Can you work these out from the model? Positions are in its coordinate system, mm. A direction names the side the tool comes from. Round coordinates to 2 decimals unless told otherwise and drop trailing zeros. Write each loop counter-clockwise with the first axis right and the second up, starting at its lowest first coordinate (ties: lowest second). Pieces come first, ordered by that corner, then holes. Notation, with made-up numbers: (43.25, -35.75) - (60.25, -35.75) arc R30 ccw to (60.25, -6.75) - close; hole circle Ø1 at (9, 22). An arc over 180 degrees is marked (long way). One line per item, written item: value. Start each with the question number.
(1) I want a section at C-C on y = 44. List the corners of the cut face in (x, z) for me, plus the area to 3 significant figures.
(2) I'm going to push flat-ended pins straight in: pin 1 Ø2 at (x, z) = (0, 15.5) entering from +Y; pin 2 Ø3 at (y, z) = (23.5, 0) entering from +X; pin 3 Ø2 at (x, y) = (-5, 17) entering from +Z. Where does each tip first touch, or does it pass through?
(3) If I drill on L1, parallel to Z at x = 0, y = 48.75; L2, parallel to Z at x = 1, y = 15.5; L3, parallel to Y at x = 0.5, z = -3, over which ranges is the centre line in solid material (lowest first)? Write a range as from..to.
(4) I want a section at A-A on y = 33. List the corners of the cut face in (x, z) for me, plus the area to 3 significant figures.
(5) I want a section at D-D on x = 0. Give the number of separate pieces and of enclosed holes in the cut face, plus the area to 3 significant figures.
(6) On a 3-axis mill with a long thin cutter (end or side, diameter ignored), from which of +Z, -Z, +X, -X, +Y, -Y can I reach the whole of each face in a straight line? I mean faces 1 (the face through (0, 43, 16)), 2 (the face through (0, 50, 0)), 3 (the face through (0, 33, -17.2)). Say none if no direction works.
(7) Thinking about a two-plate mould opening in Z: for faces 4 (the face through (-6.5, 25, -4)), 5 (the face through (0, 25, -22)), 6 (the face through (0, 7, -16)), which applies, +Z half, -Z half, draft (parallel to the pull), parting line (faces both ways), or undercut?
(8) I want a section at B-B on z = 0. List the corners of the cut face in (x, y) for me (3 decimals), plus the area to 3 significant figures.
Autodesk Inventor part; units mm, degrees
ref_plane "YZ Plane" through (0, 0, 0) normal (1, 0, 0) x (0, 1, 0)
ref_plane "XZ Plane" through (0, 0, 0) normal (0, 1, 0) x (-1, 0, 0)
ref_plane "XY Plane" through (0, 0, 0) normal (0, 0, 1) x (1, 0, 0)
sketch "Эскиз1" plane through (0, 0, 0) normal (0, 1, 0) x (-1, 0, 0)
  line L0 (6.5, 31) -> (-6.5, 31)
  line L1 (-6.5, 31) -> (-6.5, -31)
  line L2 (-6.5, -31) -> (6.5, -31)
  line L3 (6.5, -31) -> (6.5, 31)
  line L4 (-6.5, 31) -> (6.5, -31) construction
  line L5 (0, 31) -> (0, -31) construction
  circle A0 centre (0, 16) radius 2
  line L6 (6.5, 0) -> (-6.5, 0) construction
  circle A1 centre (0, -16) radius 2
  point P0 (0, 0)
  point P1 (0, 0)
  dimension "d0" = 13
  dimension "d1" = 62
  dimension "d2" = 16
  dimension "d3" = 4
extrude "Выдавливание1" add sketch "Эскиз1" along normal blind 32
sketch "Эскиз2" plane through (6.5, 0, 31) normal (1, 0, 0) x (0, 0, -1)
  line L0 (0, 32) -> (62, 32)
  line L1 (62, 0) -> (0, 0)
  line L2 (62, 32) -> (0, 0) construction
  circle A0 centre (31, 16) radius 10.15
  line L3 (20.85, 16) -> (41.15, 16) construction
  circle A1 centre (31, 16) radius 10.125
  line L4 (31, 26.125) -> (31, 5.875)
  line L5 (62, 0) -> (62, 32)
  circle A2 centre (31, 16) radius 5
  line L6 (31, 16) -> (24.504809, 12.25) construction
  line L7 (31, 16) -> (37.495191, 12.25) construction
  circle A3 centre (31, 16) radius 7.5 construction
  circle A4 centre (31, 23.5) radius 1.3
  circle A5 centre (37.495191, 12.25) radius 1.3
  circle A6 centre (24.504809, 12.25) radius 1.3
  line L8 (37.495191, 12.25) -> (36.55555, 10.622495) construction
  circle A7 centre (31, 16) radius 10 construction
  line L9 (37.495191, 12.25) -> (39.660254, 11) construction
  point P0 (31, 0)
  dimension "d60" = 20
  dimension "d9" = 20.3
  dimension "d17" = 10
  dimension "d21" = 20.25
  dimension "d57" = 120
  dimension "d58" = 120
  dimension "d59" = 2.6
  dimension "d61" = 2.5
  dimension "d65" = 15
extrude "Выдавливание3" cut sketch "Эскиз2" against normal through all contours A4 L4 | L4 A4 | A2 L4 | L4 A2 | A5 | A6
sketch "Эскиз2 outline for Выдавливание4" plane through (6.5, 0, 31) normal (1, 0, 0) x (0, 0, -1)
  circle A0 centre (31, 16) radius 10.125
extrude "Выдавливание4" cut sketch "Эскиз2 outline for Выдавливание4" against normal blind 9
sketch "Эскиз3" plane through (0, 32, 0) normal (0, 1, 0) x (1, 0, 0)
  circle A0 centre (0, -16) radius 2
  circle A1 centre (0, 16) radius 2
  point P0 (0, 0)
extrude "Выдавливание5" add sketch "Эскиз3" against normal blind 25
fillet "Сопряжение1" radius 6 2 edges at (6.5, 16, 31) (6.5, 16, -31)
chamfer "Фаска1" distance 1.3 angle 45 3 edges at (-6.5, 12.25, 7.7952) (-6.5, 12.25, -5.1952) (-6.5, 23.5, 1.3)
sketch "Эскиз6" plane through (0, 32, 0) normal (0, 1, 0) x (1, 0, 0)
  arc A0 (6.5, 25) -> (0.5, 31) centre (0.5, 25) ccw
  line L0 (0.5, 31) -> (-6.5, 31)
  line L1 (-6.5, 31) -> (-6.5, -31)
  line L2 (-6.5, -31) -> (0.5, -31)
  arc A1 (0.5, -31) -> (6.5, -25) centre (0.5, -25) ccw
  line L3 (6.5, -25) -> (6.5, 25)
  point P0 (0, 0)
extrude "Выдавливание6" add sketch "Эскиз6" along normal blind 18
sketch "Эскиз7" plane through (0, 50, 0) normal (0, 1, 0) x (1, 0, 0)
  circle A0 centre (0, -16) radius 2
  circle A1 centre (0, 16) radius 2
  point P0 (0, 0)
extrude "Выдавливание7" cut sketch "Эскиз7" against normal blind 7
sketch "Эскиз9" plane through (-6.5, 0, -31) normal (-1, 0, 0) x (0, 0, 1)
  line L0 (0, 0) -> (0, 50)
  line L1 (0, 50) -> (62, 0) construction
  line L2 (7.2, 43) -> (54.8, 43)
  line L3 (54.8, 43) -> (54.8, 7)
  line L4 (54.8, 7) -> (7.2, 7)
  line L5 (7.2, 7) -> (7.2, 43)
  line L6 (0, 50) -> (62, 50)
  line L7 (0, 0) -> (62, 0)
  line L8 (62, 0) -> (62, 50)
  line L9 (62, 0) -> (56, 0)
  line L10 (7.2, 43) -> (0, 43) construction
  line L11 (7.2, 7) -> (0, 7) construction
  line L12 (54.8, 7) -> (62, 7) construction
  line L13 (54.8, 43) -> (62, 43) construction
  arc A0 (0, 7) -> (0, 43) centre (-18.9, 25) ccw
  arc A1 (62, 43) -> (62, 7) centre (80.9, 25) ccw
  line L14 (13.8, 38.870968) -> (48.2, 38.870968) construction
  line L15 (48.2, 38.870968) -> (48.2, 26.15)
  line L16 (48.2, 26.15) -> (13.8, 26.15) construction
  line L17 (13.8, 26.15) -> (13.8, 38.870968)
  line L18 (31, 38.870968) -> (31, 50) construction
  arc A2 (48.2, 26.15) -> (13.8, 26.15) centre (31, 4.496667) ccw
  arc A3 (26.990369, 13.012884) -> (35.009631, 13.012884) centre (31, 16) ccw
  arc A4 (48.2, 37.15) -> (13.8, 37.15) centre (31, 15.496667) ccw
  line L19 (13.8, 37.15) -> (48.2, 37.15) construction
  circle A5 centre (31, 16) radius 10.15 construction
  point P0 (31, 0)
  point P1 (31, 25)
  point P2 (54.8, 25)
  point P3 (7.2, 25)
  point P4 (31, 32.15)
  dimension "d30" = 7
  dimension "d31" = 7
  dimension "d33" = 7.2
  dimension "d42" = 6.6
  dimension "d44" = 11
  dimension "d45" = 6
extrude "Выдавливание8" cut sketch "Эскиз9" against normal up to surface (13 mm away) contours L0 A0 | A1 L8
extrude "Выдавливание9" cut sketch "Эскиз9" against normal up to surface (13 mm away) contours A4 L2 | L2 A4 L15 A2 L17
fillet "Сопряжение2" radius 2 4 edges at (0, 26.15, 17.2) (0, 26.15, -17.2) (0, 37.15, 17.2) (0, 37.15, -17.2)
sketch "Эскиз11" plane through (0, 50, 0) normal (0, 1, 0) x (1, 0, 0)
  arc A0 (1, -22) -> (-3, -26) centre (1, -26) ccw
  line L0 (-3, -29.486243) -> (-3, -26)
  line L1 (5.457212, -22) -> (-4.601252, -22)
  arc A1 (-3, -29.486243) -> (-1.997801, -32.134486) centre (1, -29.486243) ccw
  arc A2 (-3, -29.486243) -> (-1.997801, -32.134486) centre (1, -29.486243) ccw
  line L2 (-1.997801, -32.134486) -> (17.505015, -54.211602)
  line L3 (6.5, -25) -> (6.5, 25)
  line L4 (5.457212, -22) -> (6.5, -22)
  arc A3 (0.5, -31) -> (6.5, -25) centre (0.5, -25) ccw
  line L5 (-6.5, -31) -> (0.5, -31)
  line L6 (6.5, -31) -> (6.5, 31)
  point P0 (0, 0)
  point P1 (-2.702505, -31)
  point P2 (-2.877907, -22)
  point P3 (0.96893, -22.000121)
extrude "Выдавливание10" cut sketch "Эскиз11" against normal up to surface (50 mm away)
mirror "Зеркальное отражение1" about plane through (0, 0, 0) normal (0, 0, 1) of "Выдавливание10"
fillet "Сопряжение3" radius 4 2 edges at (6.5, 25, 22) (6.5, 25, -22)
sketch "Эскиз12" plane through (0, 50, 0) normal (0, 1, 0) x (1, 0, 0)
  circle A0 centre (0, 16) radius 2
  circle A1 centre (0, -16) radius 2
  circle A2 centre (0, -16) radius 2
  line L0 (0, 16) -> (0, -16)
  arc A3 (6.5, 18) -> (2.5, 22) centre (2.5, 18) ccw
  line L1 (6.5, -18) -> (6.5, 18)
  arc A4 (2.5, -22) -> (6.5, -18) centre (2.5, -18) ccw
  arc A5 (-2.5, 22) -> (-6.5, 18) centre (-2.5, 18) ccw
  line L2 (-6.5, -18) -> (-6.5, 18)
  arc A6 (-6.5, -18) -> (-2.5, -22) centre (-2.5, -18) ccw
  arc A7 (6.5, 18) -> (2.5, 22) centre (2.5, 18) ccw
  line L3 (2.5, 22) -> (1, 22)
  arc A8 (-3, 26) -> (1, 22) centre (1, 26) ccw
  line L4 (-3, 26) -> (-3, 29.486243)
  arc A9 (-2.702505, 31) -> (-3, 29.486243) centre (1, 29.486243) ccw
  line L5 (-2.702505, 31) -> (-6.5, 31)
  line L6 (-6.5, 31) -> (-6.5, -31)
  line L7 (-6.5, -31) -> (-2.702505, -31)
  arc A10 (-3, -29.486243) -> (-2.702505, -31) centre (1, -29.486243) ccw
  line L8 (-3, -29.486243) -> (-3, -26)
  arc A11 (1, -22) -> (-3, -26) centre (1, -26) ccw
  line L9 (1, -22) -> (2.5, -22)
  arc A12 (2.5, -22) -> (6.5, -18) centre (2.5, -18) ccw
  line L10 (6.5, -18) -> (6.5, 18)
  circle A13 centre (0, 16) radius 2
  circle A14 centre (0, -16) radius 2
  line L11 (1, 22) -> (2.5, 22)
  line L12 (-2.5, 22) -> (2.5, 22)
  line L13 (2.5, -22) -> (1, -22)
  line L14 (-2.5, -22) -> (1, -22)
  point P0 (0, 0)
  point P1 (1, 22)
extrude "Выдавливание11" cut sketch "Эскиз12" against normal up to surface (50 mm away) contours L12 A5 L6 L5 A9 L4 A8 | A11 L8 A10 L7 L6 A6 L14
chamfer "Фаска2" distance 0.25 angle 45 8 edges at (6.5, 0, 0) (5.3284, 0, -20.8284) (0, 0, -22) (-5.3284, 0, -20.8284) (-6.5, 0, 0) (-5.3284, 0, 20.8284) (0, 0, 22) (5.3284, 0, 20.8284)
chamfer "Фаска3" distance 0.25 angle 45 8 edges at (-6.5, 43.15, 0) (-6.5, 37.0647, 16.9847) (-6.5, 33.06, 17.2) (-6.5, 28.2187, 16.1873) (-6.5, 32.15, 0) (-6.5, 28.2187, -16.1873) (-6.5, 33.06, -17.2) (-6.5, 37.0647, -16.9847)
sketch "Эскиз13" plane through (0, 0, 0) normal (0, -1, 0) x (1, 0, 0)
  point P0 (0, 0)
equation "\"d58\" = d57"
equation "\"d31\" = d30"
equation "\"Радиус_гибки\" = Толщина"
equation "\"Ширина_просечки\" = Толщина"
equation "\"Глубина_просечки\" = 0.5 * Толщина"
equation "\"Размер_просечки\" = 4 * Толщина"
equation "\"Мин_остаток\" = 2 * Толщина"
equation "\"Радиус_перехода\" = Радиус_гибки"
equation "\"Радиус_Якоби\" = Радиус_гибки"
equation "\"Размер_зазора\" = Толщина"
properties part number "motor_mount_edge_v2" material "Полиэтилен, низкая плотность"
Established:
1. outline: (-6.5, -18) arc R4 ccw to (-2.5, -22) - (2.5, -22) arc R4 ccw to (6.5, -18) - (6.5, 18) arc R4 ccw to (2.5, 22) - (-2.5, 22) arc R4 ccw to (-6.5, 18) - close; hole circle Ø4 at (0, -16); hole circle Ø4 at (0, 16)
1. area: 533 mm2
2. pin 1: y = 43
2. pin 2: x = -2.5
2. pin 3: z = 21.71
3. L1: -22..-18, -14..14, 18..22
3. L2: -22..-10.11, 10.11..22
3. L3: 0..6.33, 25.67..31.99, 42.99..50
4. outline: (-6.5, -18) arc R4 ccw to (-2.5, -22) - (2.5, -22) arc R4 ccw to (6.5, -18) - (6.5, -17.2) - (-6.25, -17.2) - (-6.5, -17.45) - close; (-6.5, 17.45) - (-6.25, 17.2) - (6.5, 17.2) - (6.5, 18) arc R4 ccw to (2.5, 22) - (-2.5, 22) arc R4 ccw to (-6.5, 18) - close
4. area: 111 mm2
5. separate pieces: 1
5. enclosed holes: 2
5. area: 1,390 mm2
6. face 1: +Y
6. face 2: +Z, -Z, +X, -X, +Y
6. face 3: +X, -X
7. face 4: draft
7. face 5: -Z half
7. face 6: undercut
8. outline: (-6.5, 0.25) - (-6.25, 0) - (6.25, 0) - (6.5, 0.25) - (6.5, 5.875) - (-2.5, 5.875) - (-2.5, 11) - (-6.5, 11) - close; (-6.5, 26.1) - (-5.2, 24.8) - (-2.5, 24.8) - (-2.5, 26.125) - (6.5, 26.125) - (6.5, 32.15) - (-6.25, 32.15) - (-6.5, 31.9) - close; (-6.5, 43.4) - (-6.25, 43.15) - (6.5, 43.15) - (6.5, 50) - (-6.5, 50) - close; (-6.4, 21) - (-2.5, 21) - (-2.5, 22.2) - (-5.2, 22.2) - close
8. area: 273 mm2
